Input: part model. Units: mm. Frame: model coordinates. Face numbers are marked on the shaded views. A direction names the side the tool comes from. Coordinates: 2 decimals unless noted, no trailing zeros. Write each loop counter-clockwise with the first axis right and the second up, starting at its lowest first coordinate (ties: lowest second). Pieces come first, ordered by that corner, then holes. Notation, with made-up numbers: (26.25, 86.5) - (70.25, 86.5) arc R20 cw to (70.25, 101.5) - close; hole circle Ø6 at (67, 52.5). An arc over 180 degrees is marked (long way). Use CSV: the item, a comma, the result in double quotes.
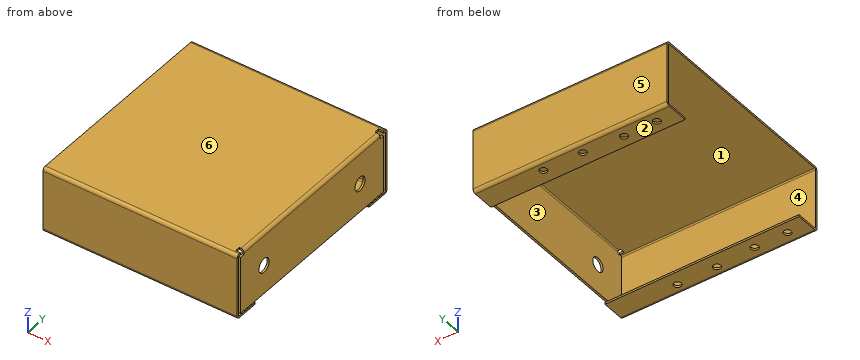
```python
from build123d import *

# Parameters (mm, degrees)
SKETCH_1_W                       = 118
SKETCH_1_H                       = 125
SM_BASE_FLANGE_1_DEPTH           = 1.2
SM_EDGE_FLANGE_2_STRIP_W         = 6.2732
SM_EDGE_FLANGE_2_STRIP_H         = 1.2
SM_EDGE_FLANGE_2_STRIP_CUT_DEPTH = 118
SM_EDGE_FLANGE_2_DEPTH           = 118
SM_EDGE_FLANGE_3_STRIP_W         = 6.2732
SM_EDGE_FLANGE_3_STRIP_H         = 1.2
SM_EDGE_FLANGE_3_STRIP_CUT_DEPTH = 118
SM_EDGE_FLANGE_3_DEPTH           = 118
SM_EDGE_FLANGE_4_STRIP_W         = 6.2732
SM_EDGE_FLANGE_4_STRIP_H         = 1.2
SM_EDGE_FLANGE_4_STRIP_CUT_DEPTH = 118
SM_EDGE_FLANGE_4_DEPTH           = 118
SM_EDGE_FLANGE_5_STRIP_W         = 6.2732
SM_EDGE_FLANGE_5_STRIP_H         = 1.2
SM_EDGE_FLANGE_5_STRIP_CUT_DEPTH = 118
SM_EDGE_FLANGE_5_DEPTH           = 118
CUT_EXTRUDE_2_REACH              = 178.491
SKETCH_22_W                      = 3
SKETCH_22_H                      = 3
SM_EDGE_FLANGE_6_STRIP_W         = 6.2732
SM_EDGE_FLANGE_6_STRIP_H         = 1.2
SM_EDGE_FLANGE_6_STRIP_CUT_DEPTH = 113.1268
SM_EDGE_FLANGE_6_DEPTH           = 113.1268
SKETCH_26_W                      = 35.0634
SKETCH_26_H                      = 3
EXTRUDE_1_DEPTH                  = 1.2
CUT_EXTRUDE_3_REACH              = 178.491
SKETCH_27_R                      = 4.25
CUT_EXTRUDE_4_REACH              = 178.491
SKETCH_28_R                      = 2.25
CUT_EXTRUDE_5_REACH              = 178.491
SKETCH_29_R                      = 2.25


# Sheet-metal steps are written as plain solids
with BuildPart() as part:
    # Sketch 1 → Базовая кромка1 (new body)
    with BuildSketch(Plane.XY):
        with Locations((59, 62.5)):
            Rectangle(SKETCH_1_W, SKETCH_1_H)
    extrude(amount=-SM_BASE_FLANGE_1_DEPTH)

    # Ребро-кромка2 strip (across the edge) → Ребро-кромка2 strip cut (cut)
    with BuildSketch(Plane(origin=(118, 0, -1.2), x_dir=(0, 1, 0), z_dir=(-1, 0, 0))):
        with Locations((-1.2, -0.6)):
            Rectangle(SM_EDGE_FLANGE_2_STRIP_W, SM_EDGE_FLANGE_2_STRIP_H)
    extrude(amount=SM_EDGE_FLANGE_2_STRIP_CUT_DEPTH, mode=Mode.SUBTRACT)

    # Ребро-кромка2 section (across the edge) → Ребро-кромка2 (add)
    with BuildSketch(Plane(origin=(118, 0, -1.2), x_dir=(0, 1, 0), z_dir=(-1, 0, 0))):
        with BuildLine():
            Line((0, 0.7366), (0, 38.8))
            Line((0, 38.8), (1.2, 38.8))
            Line((1.2, 38.8), (1.2, 0.7366))
            ThreePointArc((1.2, 0.7366), (1.415745145, 0.215745145), (1.9366, 0))
            Line((1.9366, 0), (1.9366, -1.2))
            ThreePointArc((1.9366, -1.2), (0.567217008, -0.632782992), (0, 0.7366))
        make_face()
    extrude(amount=SM_EDGE_FLANGE_2_DEPTH)

    # Ребро-кромка3 strip (across the edge) → Ребро-кромка3 strip cut (cut)
    with BuildSketch(Plane(origin=(0, 125, -1.2), x_dir=(0, -1, 0), z_dir=(1, 0, 0))):
        with Locations((-1.2, -0.6)):
            Rectangle(SM_EDGE_FLANGE_3_STRIP_W, SM_EDGE_FLANGE_3_STRIP_H)
    extrude(amount=SM_EDGE_FLANGE_3_STRIP_CUT_DEPTH, mode=Mode.SUBTRACT)

    # Ребро-кромка3 section (across the edge) → Ребро-кромка3 (add)
    with BuildSketch(Plane(origin=(0, 125, -1.2), x_dir=(0, -1, 0), z_dir=(1, 0, 0))):
        with BuildLine():
            Line((0, 0.7366), (0, 38.8))
            Line((0, 38.8), (1.2, 38.8))
            Line((1.2, 38.8), (1.2, 0.7366))
            ThreePointArc((1.2, 0.7366), (1.415745145, 0.215745145), (1.9366, 0))
            Line((1.9366, 0), (1.9366, -1.2))
            ThreePointArc((1.9366, -1.2), (0.567217008, -0.632782992), (0, 0.7366))
        make_face()
    extrude(amount=SM_EDGE_FLANGE_3_DEPTH)

    # Ребро-кромка4 strip (across the edge) → Ребро-кромка4 strip cut (cut)
    with BuildSketch(Plane(origin=(0, 123.8, -40), x_dir=(0, 0, 1), z_dir=(1, 0, 0))):
        with Locations((-1.2, -0.6)):
            Rectangle(SM_EDGE_FLANGE_4_STRIP_W, SM_EDGE_FLANGE_4_STRIP_H)
    extrude(amount=SM_EDGE_FLANGE_4_STRIP_CUT_DEPTH, mode=Mode.SUBTRACT)

    # Ребро-кромка4 section (across the edge) → Ребро-кромка4 (add)
    with BuildSketch(Plane(origin=(0, 123.8, -40), x_dir=(0, 0, 1), z_dir=(1, 0, 0))):
        with BuildLine():
            Line((0, 0.7366), (0, 13.8))
            Line((0, 13.8), (1.2, 13.8))
            Line((1.2, 13.8), (1.2, 0.7366))
            ThreePointArc((1.2, 0.7366), (1.415745145, 0.215745145), (1.9366, 0))
            Line((1.9366, 0), (1.9366, -1.2))
            ThreePointArc((1.9366, -1.2), (0.567217008, -0.632782992), (0, 0.7366))
        make_face()
    extrude(amount=SM_EDGE_FLANGE_4_DEPTH)

    # Ребро-кромка5 strip (across the edge) → Ребро-кромка5 strip cut (cut)
    with BuildSketch(Plane(origin=(118, 1.2, -40), x_dir=(0, 0, 1), z_dir=(-1, 0, 0))):
        with Locations((-1.2, -0.6)):
            Rectangle(SM_EDGE_FLANGE_5_STRIP_W, SM_EDGE_FLANGE_5_STRIP_H)
    extrude(amount=SM_EDGE_FLANGE_5_STRIP_CUT_DEPTH, mode=Mode.SUBTRACT)

    # Ребро-кромка5 section (across the edge) → Ребро-кромка5 (add)
    with BuildSketch(Plane(origin=(118, 1.2, -40), x_dir=(0, 0, 1), z_dir=(-1, 0, 0))):
        with BuildLine():
            Line((0, 0.7366), (0, 13.8))
            Line((0, 13.8), (1.2, 13.8))
            Line((1.2, 13.8), (1.2, 0.7366))
            ThreePointArc((1.2, 0.7366), (1.415745145, 0.215745145), (1.9366, 0))
            Line((1.9366, 0), (1.9366, -1.2))
            ThreePointArc((1.9366, -1.2), (0.567217008, -0.632782992), (0, 0.7366))
        make_face()
    extrude(amount=SM_EDGE_FLANGE_5_DEPTH)

    # Эскиз22 → Вырез-Вытянуть2 (cut, up to next)
    with BuildSketch(Plane.XY, mode=Mode.PRIVATE) as cut_extrude_2_sk1:
        with Locations((116.5, 120.5634)):
            Rectangle(SKETCH_22_W, SKETCH_22_H)
    cut_extrude_2_tool1 = extrude(cut_extrude_2_sk1.sketch, amount=-CUT_EXTRUDE_2_REACH, mode=Mode.PRIVATE) & part.part
    # Эскиз22 → Вырез-Вытянуть2 (cut, up to next)
    with BuildSketch(Plane.XY, mode=Mode.PRIVATE) as cut_extrude_2_sk2:
        with Locations((116.5, 4.4366)):
            Rectangle(SKETCH_22_W, SKETCH_22_H)
    cut_extrude_2_tool2 = extrude(cut_extrude_2_sk2.sketch, amount=-CUT_EXTRUDE_2_REACH, mode=Mode.PRIVATE) & part.part
    add(cut_extrude_2_tool1.solids().sort_by_distance((116.5, 120.5634, 0))[0], mode=Mode.SUBTRACT)
    add(cut_extrude_2_tool2.solids().sort_by_distance((116.5, 4.4366, 0))[0], mode=Mode.SUBTRACT)

    # Ребро-кромка6 strip (across the edge) → Ребро-кромка6 strip cut (cut)
    with BuildSketch(Plane(origin=(118, 119.0634, -1.2), x_dir=(-1, 0, 0), z_dir=(0, -1, 0))):
        with Locations((-1.2, -0.6)):
            Rectangle(SM_EDGE_FLANGE_6_STRIP_W, SM_EDGE_FLANGE_6_STRIP_H)
    extrude(amount=SM_EDGE_FLANGE_6_STRIP_CUT_DEPTH, mode=Mode.SUBTRACT)

    # Ребро-кромка6 section (across the edge) → Ребро-кромка6 (add)
    with BuildSketch(Plane(origin=(118, 119.0634, -1.2), x_dir=(-1, 0, 0), z_dir=(0, -1, 0))):
        with BuildLine():
            Line((0, 0.7366), (0, 36.8))
            Line((0, 36.8), (1.2, 36.8))
            Line((1.2, 36.8), (1.2, 0.7366))
            ThreePointArc((1.2, 0.7366), (1.415745145, 0.215745145), (1.9366, 0))
            Line((1.9366, 0), (1.9366, -1.2))
            ThreePointArc((1.9366, -1.2), (0.567217008, -0.632782992), (0, 0.7366))
        make_face()
    extrude(amount=SM_EDGE_FLANGE_6_DEPTH)

    # Эскиз26 → Бобышка-Вытянуть1 (add)
    with BuildSketch(Plane(origin=(118, 0, 0), x_dir=(0, 0, -1), z_dir=(1, 0, 0))):
        with Locations((20.4683, 120.5634)):
            Rectangle(SKETCH_26_W, SKETCH_26_H)
        with Locations((20.4683, 4.4366)):
            Rectangle(SKETCH_26_W, SKETCH_26_H)
    extrude(amount=-EXTRUDE_1_DEPTH)

    # Эскиз27 → Вырез-Вытянуть3 (cut, up to next)
    with BuildSketch(Plane(origin=(118, 0, 0), x_dir=(0, 0, -1), z_dir=(1, 0, 0)), mode=Mode.PRIVATE) as cut_extrude_3_sk1:
        with Locations((20.4683, 102.5)):
            Circle(SKETCH_27_R)
    cut_extrude_3_tool1 = extrude(cut_extrude_3_sk1.sketch, amount=-CUT_EXTRUDE_3_REACH, mode=Mode.PRIVATE) & part.part
    # Эскиз27 → Вырез-Вытянуть3 (cut, up to next)
    with BuildSketch(Plane(origin=(118, 0, 0), x_dir=(0, 0, -1), z_dir=(1, 0, 0)), mode=Mode.PRIVATE) as cut_extrude_3_sk2:
        with Locations((20.4683, 22.5)):
            Circle(SKETCH_27_R)
    cut_extrude_3_tool2 = extrude(cut_extrude_3_sk2.sketch, amount=-CUT_EXTRUDE_3_REACH, mode=Mode.PRIVATE) & part.part
    add(cut_extrude_3_tool1.solids().sort_by_distance((118, 102.5, -20.4683))[0], mode=Mode.SUBTRACT)
    add(cut_extrude_3_tool2.solids().sort_by_distance((118, 22.5, -20.4683))[0], mode=Mode.SUBTRACT)

    # Эскиз28 → Вырез-Вытянуть4 (cut, up to next)
    with BuildSketch(Plane(origin=(0, 0, -40), x_dir=(-1, 0, 0), z_dir=(0, 0, -1)), mode=Mode.PRIVATE) as cut_extrude_4_sk1:
        with Locations(Location((-80, 118.4683, 0), (0, 0, 90))):
            Circle(SKETCH_28_R)
    cut_extrude_4_tool1 = extrude(cut_extrude_4_sk1.sketch, amount=-CUT_EXTRUDE_4_REACH, mode=Mode.PRIVATE) & part.part
    # Эскиз28 → Вырез-Вытянуть4 (cut, up to next)
    with BuildSketch(Plane(origin=(0, 0, -40), x_dir=(-1, 0, 0), z_dir=(0, 0, -1)), mode=Mode.PRIVATE) as cut_extrude_4_sk2:
        with Locations(Location((-56, 118.4683, 0), (0, 0, 90))):
            Circle(SKETCH_28_R)
    cut_extrude_4_tool2 = extrude(cut_extrude_4_sk2.sketch, amount=-CUT_EXTRUDE_4_REACH, mode=Mode.PRIVATE) & part.part
    # Эскиз28 → Вырез-Вытянуть4 (cut, up to next)
    with BuildSketch(Plane(origin=(0, 0, -40), x_dir=(-1, 0, 0), z_dir=(0, 0, -1)), mode=Mode.PRIVATE) as cut_extrude_4_sk3:
        with Locations(Location((-80, 6.5317, 0), (0, 0, 90))):
            Circle(SKETCH_28_R)
    cut_extrude_4_tool3 = extrude(cut_extrude_4_sk3.sketch, amount=-CUT_EXTRUDE_4_REACH, mode=Mode.PRIVATE) & part.part
    # Эскиз28 → Вырез-Вытянуть4 (cut, up to next)
    with BuildSketch(Plane(origin=(0, 0, -40), x_dir=(-1, 0, 0), z_dir=(0, 0, -1)), mode=Mode.PRIVATE) as cut_extrude_4_sk4:
        with Locations(Location((-56, 6.5317, 0), (0, 0, 90))):
            Circle(SKETCH_28_R)
    cut_extrude_4_tool4 = extrude(cut_extrude_4_sk4.sketch, amount=-CUT_EXTRUDE_4_REACH, mode=Mode.PRIVATE) & part.part
    add(cut_extrude_4_tool1.solids().sort_by_distance((80, 118.4683, -40))[0], mode=Mode.SUBTRACT)
    add(cut_extrude_4_tool2.solids().sort_by_distance((56, 118.4683, -40))[0], mode=Mode.SUBTRACT)
    add(cut_extrude_4_tool3.solids().sort_by_distance((80, 6.5317, -40))[0], mode=Mode.SUBTRACT)
    add(cut_extrude_4_tool4.solids().sort_by_distance((56, 6.5317, -40))[0], mode=Mode.SUBTRACT)

    # Эскиз29 → Вырез-Вытянуть5 (cut, up to next)
    with BuildSketch(Plane(origin=(0, 0, -40), x_dir=(-1, 0, 0), z_dir=(0, 0, -1)), mode=Mode.PRIVATE) as cut_extrude_5_sk1:
        with Locations(Location((-32, 117, 0), (0, 0, 90))):
            Circle(SKETCH_29_R)
    cut_extrude_5_tool1 = extrude(cut_extrude_5_sk1.sketch, amount=-CUT_EXTRUDE_5_REACH, mode=Mode.PRIVATE) & part.part
    # Эскиз29 → Вырез-Вытянуть5 (cut, up to next)
    with BuildSketch(Plane(origin=(0, 0, -40), x_dir=(-1, 0, 0), z_dir=(0, 0, -1)), mode=Mode.PRIVATE) as cut_extrude_5_sk2:
        with Locations(Location((-12, 117, 0), (0, 0, 90))):
            Circle(SKETCH_29_R)
    cut_extrude_5_tool2 = extrude(cut_extrude_5_sk2.sketch, amount=-CUT_EXTRUDE_5_REACH, mode=Mode.PRIVATE) & part.part
    # Эскиз29 → Вырез-Вытянуть5 (cut, up to next)
    with BuildSketch(Plane(origin=(0, 0, -40), x_dir=(-1, 0, 0), z_dir=(0, 0, -1)), mode=Mode.PRIVATE) as cut_extrude_5_sk3:
        with Locations(Location((-32, 8, 0), (0, 0, 90))):
            Circle(SKETCH_29_R)
    cut_extrude_5_tool3 = extrude(cut_extrude_5_sk3.sketch, amount=-CUT_EXTRUDE_5_REACH, mode=Mode.PRIVATE) & part.part
    # Эскиз29 → Вырез-Вытянуть5 (cut, up to next)
    with BuildSketch(Plane(origin=(0, 0, -40), x_dir=(-1, 0, 0), z_dir=(0, 0, -1)), mode=Mode.PRIVATE) as cut_extrude_5_sk4:
        with Locations(Location((-12, 8, 0), (0, 0, 90))):
            Circle(SKETCH_29_R)
    cut_extrude_5_tool4 = extrude(cut_extrude_5_sk4.sketch, amount=-CUT_EXTRUDE_5_REACH, mode=Mode.PRIVATE) & part.part
    add(cut_extrude_5_tool1.solids().sort_by_distance((32, 117, -40))[0], mode=Mode.SUBTRACT)
    add(cut_extrude_5_tool2.solids().sort_by_distance((12, 117, -40))[0], mode=Mode.SUBTRACT)
    add(cut_extrude_5_tool3.solids().sort_by_distance((32, 8, -40))[0], mode=Mode.SUBTRACT)
    add(cut_extrude_5_tool4.solids().sort_by_distance((12, 8, -40))[0], mode=Mode.SUBTRACT)


solid = part.part
```
(1) Ray query, probe 1 along Y at (x, z) = (15, -27.5); probe 2 along Z at (x, y) = (104.5, 13); probe 3 along X at (y, z) = (117, -39.25). Return the intervals inside material, ascending. Write a range as from..to.
Check values:
probe 1,"0..1.2, 123.8..125"
probe 2,"-40..-38.8, -1.2..0"
probe 3,"0..9.75, 14.25..29.75, 34.25..54.3, 57.7..78.3, 81.7..118"
(2) Draft query along Z for the marked faces 3, 4, 5 and 6. Return one class per face: pulls with the +Z half, pulls with the -Z half, needs draft (parallel to the pull), parting line crosses it, or undercut.
Check values:
face 3,"undercut"
face 4,"undercut"
face 5,"needs draft"
face 6,"pulls with the +Z half"
(3) Reachability of the marked faces 1 and 2 from +Z, -Z, +X, -X, +Y, -Y: full face, straight path, thin tool, end or side. Return the list, or none.
Check values:
face 1,"-X"
face 2,"-Z, +X, -X, +Y, -Y"
(4) Cut plane B-B on x = 56. Return loops of the section in (y, z), and give its area (3 significant figures).
Check values:
outline,"(0, -38.06) arc R1.94 ccw to (1.94, -40) - (4.28, -40) - (4.28, -38.8) - (1.94, -38.8) arc R0.74 cw to (1.2, -38.06) - (1.2, -1.94) arc R0.74 cw to (1.94, -1.2) - (123.06, -1.2) arc R0.74 cw to (123.8, -1.94) - (123.8, -38.06) arc R0.74 cw to (123.06, -38.8) - (120.72, -38.8) - (120.72, -40) - (123.06, -40) arc R1.94 ccw to (125, -38.06) - (125, -1.94) arc R1.94 ccw to (123.06, 0) - (1.94, 0) arc R1.94 ccw to (0, -1.94) - close; (8.78, -40) - (15, -40) - (15, -38.8) - (8.78, -38.8) - close; (110, -40) - (116.22, -40) - (116.22, -38.8) - (110, -38.8) - close"
area,"263 mm^2"
(5) Cut plane A-A on z = -13.5. Return loops of the section in (x, y).
Check values:
outline,"(0, 0) - (118, 0) - (118, 1.2) - (0, 1.2) - close; (0, 123.8) - (118, 123.8) - (118, 125) - (0, 125) - close; (116.8, 2.94) - (118, 2.94) - (118, 122.06) - (116.8, 122.06) - close"
(6) Pin query (flat end, axial travel): pin 1 Ø4 at (x, y) = (43, 115.5) entering from +Z; pin 2 Ø2 at (x, y) = (91, 22) entering from -Z; pin 3 Ø0.6 at (y, z) = (121, -0.5) entering from +X; pin 4 Ø10 at (y, z) = (102.5, -20.47) entering from -X. Return the tip coordinate at first contact, or that it passes through.
Check values:
pin 1,"z = 0"
pin 2,"z = -1.2"
pin 3,"x = 115"
pin 4,"x = 116.8"
(7) Cut plane D-D on y = 92. Return loops of the section in (x, z).
Check values:
outline,"(0, -1.2) - (116.06, -1.2) arc R0.74 cw to (116.8, -1.94) - (116.8, -38) - (118, -38) - (118, -1.94) arc R1.94 ccw to (116.06, 0) - (0, 0) - close"
(8) Cut plane C-C on y = 22.5. Return loops of the section in (x, z), and give its area (3 significant figures).
Check values:
outline,"(0, -1.2) - (116.06, -1.2) arc R0.74 cw to (116.8, -1.94) - (116.8, -16.22) - (118, -16.22) - (118, -1.94) arc R1.94 ccw to (116.06, 0) - (0, 0) - close; (116.8, -38) - (118, -38) - (118, -24.72) - (116.8, -24.72) - close"
area,"175 mm^2"
